Here's how the part is built. I have some questions about the finished solid (model axes, mm). A direction names the side the tool comes from. Give positions to 0.01 mm unless a question says otherwise; leave off trailing zeros. Write each loop counter-clockwise with the first axis right and the second up, starting at its lowest first coordinate (ties: lowest second). Pieces come first, ordered by that corner, then holes. Notation, with made-up numbers: M 44.25,55 L 75.25,55 A15 cw 75.25,78 Z; hole C 35.25,21.5 d3. An arc over 180 degrees is marked long. Use one line per item in the form item = value. Start each with the question number.
from build123d import *

# Parameters (mm, degrees)
F0_W     = 41.372892
F0_H     = 35.991504
F1_DEPTH = 101.6
F2_DEPTH = 76.2


with BuildPart() as f1:
    # F0 (on Top) → F1 (new body)
    with BuildSketch(Plane.XY):
        Rectangle(F0_W, F0_H)
    extrude(amount=F1_DEPTH)

    # F0 (on Top) → F2 (join)
    with BuildSketch(Plane.XY):
        with BuildLine():
            Line((-20.686446, 17.995752), (20.686446, 17.995752))
            ThreePointArc((20.686446, 17.995752), (0, 27.418536), (-20.686446, 17.995752))
        make_face()
        with BuildLine():
            Line((-20.686446, -17.995752), (-20.686446, 17.995752))
            ThreePointArc((-20.686446, 17.995752), (-27.418536, 0), (-20.686446, -17.995752))
        make_face()
        with BuildLine():
            ThreePointArc((-20.686446, -17.995752), (0, -27.418536), (20.686446, -17.995752))
            Line((20.686446, -17.995752), (-20.686446, -17.995752))
        make_face()
    extrude(amount=F2_DEPTH)


solid = f1.part
1) Suppose I cut it at C-C, the plane y = 14. List the corners of the cut face in (x, z) for me, and give its area (3 significant figures).
2) Suppose I cut it at A-A, the plane x = 0. List the corners of the cut face in (y, z) for me.
3) On a 3-axis mill with a long thin cutter (end or side, diameter ignored), from which of +Z, -Z, +X, -X, +Y, -Y can I reach the whole of each face in a straight line? I mean faces 1 (the face through (0, -22, 76.2)), 2 (the face through (0, 22, 76.2)), 3 (the face through (-20.686, 0, 89)). Say none if no direction works.
4) Suppose I cut it at D-D, the plane x = 10. List the corners of the cut face in (y, z) for me.
5) Please list where these lines run through material, in increasing order: line 1 (X direction, y = 14.5, z = 81.5); line 2 (Y direction, x = -16.5, z = 96.5); line 3 (Z direction, x = -21, y = -7.5).
6) Will these pins go through, and if not, where does the flat tip stop? P1, Ø4, axis at x = -20.5, z = 13, coming from the +Y side; P2, Ø2, axis at x = -13.5, z = 44.5, coming from the +Y side; P3, Ø7.5, axis at x = -4.5, y = 22.5, coming from the +Z side.
7) Suppose I cut it at B-B, the plane z = 40. List the corners of the cut face in (x, y) for me, and give its area (3 significant figures).
Checks:
q1.outline = M -23.57,0 L 20.69,0 L 20.69,101.6 L -20.69,101.6 L -20.69,76.2 L -23.57,76.2 Z
q1.area = 4,420 mm^2
q2.outline = M -27.42,0 L 27.42,0 L 27.42,76.2 L 18,76.2 L 18,101.6 L -18,101.6 L -18,76.2 L -27.42,76.2 Z
q3.face_1 = +Z, +X, -X, -Y
q3.face_2 = +Z, +X, -X, +Y
q3.face_3 = +Z, -X, +Y, -Y
q4.outline = M -25.53,0 L 25.53,0 L 25.53,76.2 L 18,76.2 L 18,101.6 L -18,101.6 L -18,76.2 L -25.53,76.2 Z
q5.line_1 = -20.69 to 20.69
q5.line_2 = -18 to 18
q5.line_3 = 0 to 76.2
q6.P1 = 20.24
q6.P2 = 24.4
q6.P3 = 76.2
q7.outline = M -20.69,-18 A27.42 ccw 20.69,-18 L 20.69,18 A27.42 ccw -20.69,18 A27.42 ccw Z
q7.area = 2,200 mm^2
